```python
from build123d import *

# Parameters (mm, degrees)
CUT_EXTRUDE1_DEPTH = 10
CIRPATTERN1_COUNT  = 3


with BuildPart() as part:
    # Sketch1 → Revolve1 (revolve)
    with BuildSketch(Plane.XY):
        Polygon((-0.5, -38), (-0.5, 38), (-3.5, 38), (-3.5, -23.32914466), (-3.5, -38), align=None)
    revolve(axis=Axis((3.5, 38, 0), (0, -1, 0)))

    # Sketch3 → Cut-Extrude1 (cut)
    with BuildSketch(Plane.XY):
        with BuildLine():
            Line((1, 21.251316376), (1, 29.251316376))
            ThreePointArc((1, 29.251316376), (3.5, 31.751316376), (6, 29.251316376))
            Line((6, 29.251316376), (6, 21.251316376))
            ThreePointArc((6, 21.251316376), (3.5, 18.751316376), (1, 21.251316376))
        make_face()
        with BuildLine():
            Line((6.5, 4.25), (6.5, -3.75))
            ThreePointArc((6.5, -3.75), (3.5, -6.75), (0.5, -3.75))
            Line((0.5, -3.75), (0.5, 4.25))
            ThreePointArc((0.5, 4.25), (3.5, 7.25), (6.5, 4.25))
        make_face()
    cut_extrude1 = extrude(amount=-CUT_EXTRUDE1_DEPTH, mode=Mode.SUBTRACT)

    # CirPattern1: Cut-Extrude1 ×3 about axis
    cirpattern1_axis = Axis((3.5, 0, 0), (0, 1, 0))
    for i in range(1, CIRPATTERN1_COUNT):
        add(cut_extrude1.rotate(cirpattern1_axis, i * 360 / CIRPATTERN1_COUNT), mode=Mode.SUBTRACT)


solid = part.part
```
Geometry: final body of the model. Coordinates: model frame, mm. A direction names the side the tool comes from. Coordinates: 2 decimals unless noted, no trailing zeros. Order: outer loops, then holes, each group sorted by start corner. A loop starts at its lowest first (then second) coordinate and runs counter-clockwise, first axis right, second up. Notation, with made-up numbers: (74, 36) -> (110, 36) arc R21 cw to (110, 53) -> close; hole circle Ø9 at (-32.5, 65.5). An arc over 180 degrees is marked (long way). Write item = value, one per line.
(1) Cut plane A-A on y = 3.5. Return loops of the section in (x, z).
Solved:
outline = (-3.48, 0.56) arc R7 ccw to (0.5, -6.32) -> (0.5, -2.65) arc R4 cw to (-0.29, -1.28) -> close; (-0.48, 5.76) -> (2.71, 3.92) arc R4 cw to (4.29, 3.92) -> (7.48, 5.76) arc R7 ccw to start; (6.5, -6.32) arc R7 ccw to (10.48, 0.56) -> (7.29, -1.28) arc R4 cw to (6.5, -2.65) -> close
(2) Cut plane B-B on x = 3.5. Return loops of the section in (y, z), plus the area to 3 significant figures.
Solved:
outline = (-38, -7) -> (-6.75, -7) -> (-6.75, -4) -> (-38, -4) -> close; (-38, 4) -> (38, 4) -> (38, 7) -> (-38, 7) -> close; (7.25, -7) -> (18.75, -7) -> (18.75, -4) -> (7.25, -4) -> close; (31.75, -7) -> (38, -7) -> (38, -4) -> (31.75, -4) -> close
area = 375 mm²
(3) Access query for faces 3 (the cylindrical face through (7.89, 31.75, 2.47)), 4 (the flat face through (6.413, 25.307, 4.568)), 5 (the flat face through (0.587, 25.195, 4.568)). Directions: +Z, -Z, +X, -X, +Y, -Y. A direction counts if a zero-diameter tool reaches every point of the face in a straight line with its end or side. Return the directions, or none.
Solved:
face_3 = none
face_4 = +X
face_5 = -X
(4) Cut plane C-C on y = -25.5. Return loops of the section in (x, z).
Solved:
outline = circle Ø14 at (3.5, 0); hole circle Ø8 at (3.5, 0)
(5) Line query: line 1 (X direction, y = 7, z = 0); line 2 (Z direction, x = 3.5, y = 15); line 3 (Z direction, x = 6.75, y = 7.5). Output: solid intervals per line, ascending.
Solved:
line_1 = -3.5 to -0.5, 7.5 to 10.5
line_2 = -7 to -4, 4 to 7
line_3 = -6.2 to -2.33, 2.33 to 6.2
(6) Pin query (flat end, axial travel): pin 1 Ø3 at (y, z) = (0.5, -4.5) entering from +X; pin 2 Ø1 at (y, z) = (27, -5.5) entering from -X; pin 3 Ø2.5 at (y, z) = (23.5, -5.5) entering from +X. Return the tip coordinate at first contact, or that it passes through.
Solved:
pin_1 = 9.82
pin_2 = -1.4
pin_3 = 9.06
(7) Pull-direction query (Y, two-part tool) for faces 1 (the cylindrical face through (3.55, 18.75, -5.04)), 2 (the flat face through (0, -38, 3)); classes: pulls with the +Y half, pulls with the -Y half, needs draft (parallel to the pull), parting line crosses it, or undercut.
Solved:
face_1 = undercut
face_2 = pulls with the -Y half
